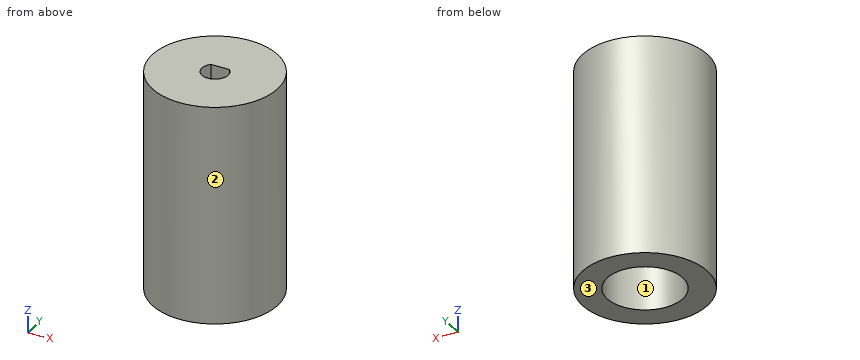
```python
from build123d import *

# Parameters (mm, degrees)
ESQUISSE1_R             = 10
ESQUISSE1_R_2           = 6.05
BOSS_EXTRU_1_DEPTH      = 35
ESQUISSE1_3_R           = 6.05
ENL_V_MAT_EXTRU_1_DEPTH = 25
ENL_V_MAT_EXTRU_2_DEPTH = 9


with BuildPart() as part:
    # Esquisse1 → Boss.-Extru.1 (new body)
    # profile 1 of 2: a face of its own
    with BuildSketch(Plane.XY):
        Circle(ESQUISSE1_R)
        Circle(ESQUISSE1_R_2, mode=Mode.SUBTRACT)
    # profile 2 of 2: a face of its own
    with BuildSketch(Plane.XY):
        Circle(ESQUISSE1_R_2)
    extrude(amount=BOSS_EXTRU_1_DEPTH)

    # Esquisse1_3 → Enl_v. mat.-Extru.1 (cut)
    with BuildSketch(Plane.XY):
        Circle(ESQUISSE1_3_R)
    extrude(amount=ENL_V_MAT_EXTRU_1_DEPTH, mode=Mode.SUBTRACT)

    # Esquisse2 → Enl_v. mat.-Extru.2 (cut)
    with BuildSketch(Plane.XY.offset(35)):
        with BuildLine():
            Line((-1.469693846, 1.5), (1.469693846, 1.5))
            ThreePointArc((1.469693846, 1.5), (0, -2.1), (-1.469693846, 1.5))
        make_face()
    extrude(amount=-ENL_V_MAT_EXTRU_2_DEPTH, mode=Mode.SUBTRACT)


solid = part.part
```
Check sheet for the modelled part. Datum: model origin and axes. Units: mm. Face numbers are marked on the shaded views. Give positions to 0.01 mm unless a question says otherwise; leave off trailing zeros. Order: outer loops, then holes, each group sorted by start corner. A loop starts at its lowest first (then second) coordinate and runs counter-clockwise, first axis right, second up. Notation, with made-up numbers: (6, 43) -> (47, 43) arc R19 ccw to (47, 56) -> close; hole circle Ø2 at (8.25, -12). An arc over 180 degrees is marked (long way). Use CSV: the item, a comma, the result in double quotes. Start each with the question number.
1) Sectioned sample at B-B, the plane y = 0. Record the boundary of the cut face in (x, z).
2) Sectioned sample at A-A, the plane x = 0. Record the boundary of the cut face in (y, z), plus the area to 3 significant figures.
3) Sectioned sample at D-D, the plane x = -5.5. Record the boundary of the cut face in (y, z), plus the area to 3 significant figures.
4) Sectioned sample at C-C, the plane z = 20.5. Record the boundary of the cut face in (x, y).
5) Material ranges on line 1 (Y direction, x = 0, z = 29); line 2 (Y direction, x = 0, z = 9.25); line 3 (Z direction, x = 3, y = 2.75), recorded low to high. Write a range as from..to.
6) Go/stop test with flat-tipped pins: P1, Ø1.1, axis at x = 0.5, y = -0.5, coming from the +Z side; P2, Ø6.5, axis at x = 0, y = 0, coming from the -Z side; P3, Ø12, axis at y = 6.5, z = 8, coming from the -X side. Record where each tip stops, or that it passes through.
7) Mould release check, pull along X, two halves, no side actions. Record for the marked faces 1, 2 and 3: released by +X, released by -X, zero draft, split by the parting line, or undercut.
Recorded:
1,outline,"(-10, 0) -> (-6.05, 0) -> (-6.05, 25) -> (6.05, 25) -> (6.05, 0) -> (10, 0) -> (10, 35) -> (2.1, 35) -> (2.1, 26) -> (-2.1, 26) -> (-2.1, 35) -> (-10, 35) -> close"
2,outline,"(-10, 0) -> (-6.05, 0) -> (-6.05, 25) -> (6.05, 25) -> (6.05, 0) -> (10, 0) -> (10, 35) -> (1.5, 35) -> (1.5, 26) -> (-2.1, 26) -> (-2.1, 35) -> (-10, 35) -> close"
2,area,"365 mm2"
3,outline,"(-8.35, 0) -> (-2.52, 0) -> (-2.52, 25) -> (2.52, 25) -> (2.52, 0) -> (8.35, 0) -> (8.35, 35) -> (-8.35, 35) -> close"
3,area,"459 mm2"
4,outline,"circle Ø20 at (0, 0); hole circle Ø12.1 at (0, 0)"
5,line 1,"-10..-2.1, 1.5..10"
5,line 2,"-10..-6.05, 6.05..10"
5,line 3,"25..35"
6,P1,"z = 26"
6,P2,"z = 25"
6,P3,"x = -9.99"
7,face 1,"undercut"
7,face 2,"split by the parting line"
7,face 3,"zero draft"
